```python
from build123d import *

# Parameters (mm, degrees)
BOSS_EXTRUDE1_DEPTH = 3
SKETCH2_R           = 2.5
SKETCH2_R_2         = 1.5
BOSS_EXTRUDE2_DEPTH = 5


with BuildPart() as part:
    # Sketch3 → Boss-Extrude1 (new body)
    with BuildSketch(Plane.XY):
        with BuildLine():
            Line((0, -4.8), (12, -4.8))
            Line((12, -4.8), (12, 4.8))
            Line((12, 4.8), (0, 4.8))
            ThreePointArc((0, 4.8), (-4.8, 0), (0, -4.8))
        make_face()
    extrude(amount=BOSS_EXTRUDE1_DEPTH)

    # Sketch2 → Boss-Extrude2 (add)
    with BuildSketch(Plane.XY):
        Circle(SKETCH2_R)
        with Locations((8.4, 0)):
            Circle(SKETCH2_R_2)
    extrude(amount=BOSS_EXTRUDE2_DEPTH)


solid = part.part
```
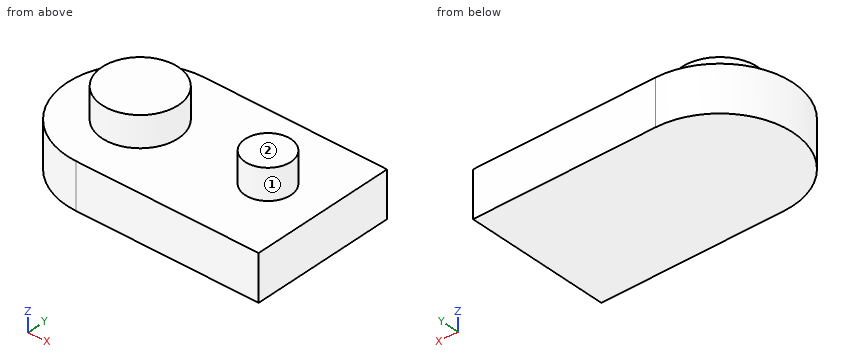
Here's how the part is built. I have some questions about the finished solid (model axes, mm). Face numbers are marked on the shaded views. A direction names the side the tool comes from. Give positions to 0.01 mm unless a question says otherwise; leave off trailing zeros. Order: outer loops, then holes, each group sorted by start corner. A loop starts at its lowest first (then second) coordinate and runs counter-clockwise, first axis right, second up. Notation, with made-up numbers: M 53.25,-1 L 75.25,-1 A32 cw 75.25,30 Z; hole C 67.5,39 d4. An arc over 180 degrees is marked long. Use a Markdown table: item, result. Add a question column.
1. Suppose I cut it at C-C (z = 3.65). List the corners of the cut face in (x, y) for me.
2. Suppose I cut it at D-D (z = 2). List the corners of the cut face in (x, y) for me, and give its area (3 significant figures).
3. On a 3-axis mill with a long thin cutter (end or side, diameter ignored), from which of +Z, -Z, +X, -X, +Y, -Y can I reach the whole of each face in a straight line? I mean the marked faces 1 and 2. Say none if no direction works.
4. I need wall thicknesses on probe 1 along Z at (x, y) = (2.75, -3.25); probe 2 along X at (y, z) = (-0.25, 3.2); probe 3 along X at (y, z) = (-0.5, 3.95). Which ranges of each line are inside material? Lowest first, please. Write a range as from..to.
5. Suppose I cut it at B-B (x = 2). List the corners of the cut face in (y, z) for me, and give its area (3 significant figures).
6. Suppose I cut it at A-A (y = 0). List the corners of the cut face in (x, z) for me.
Results list:
| question | item | result |
|---|---|---|
| 1 | outline | C 0,0 d5; C 8.4,0 d3 |
| 2 | outline | M 0,-4.8 L 12,-4.8 L 12,4.8 L 0,4.8 A4.8 ccw Z |
| 2 | area | 151 mm² |
| 3 | face 1 | +Z |
| 3 | face 2 | +Z, +X, -X, +Y, -Y |
| 4 | probe 1 | z = 0..3 |
| 4 | probe 2 | x = -2.49..2.49, 6.92..9.88 |
| 4 | probe 3 | x = -2.45..2.45, 6.99..9.81 |
| 5 | outline | M -4.8,0 L 4.8,0 L 4.8,3 L 1.5,3 L 1.5,5 L -1.5,5 L -1.5,3 L -4.8,3 Z |
| 5 | area | 34.8 mm² |
| 6 | outline | M -4.8,0 L 12,0 L 12,3 L 9.9,3 L 9.9,5 L 6.9,5 L 6.9,3 L 2.5,3 L 2.5,5 L -2.5,5 L -2.5,3 L -4.8,3 Z |
